Work out the finished part from the listing and answer in its coordinate system (mm). Face numbers are marked on the shaded views. Coordinates: 2 decimals unless noted, no trailing zeros. Write each loop counter-clockwise with the first axis right and the second up, starting at its lowest first coordinate (ties: lowest second). Pieces come first, ordered by that corner, then holes. Notation, with made-up numbers: (-28, 70) - (14, 70) arc R20 cw to (14, 91) - close; hole circle Ø6 at (52.25, 85). An arc over 180 degrees is marked (long way). One line per item, written item: value.
Autodesk Inventor part; units mm, degrees
ref_plane "center_point_XY" through (4.5, 0, 0) normal (1, 0, 0) x (0, 0, -1)
ref_plane "center_point_YZ" through (4.5, 0, 0) normal (0, 0, -1) x (0, 1, 0)
ref_plane "center_point_ZX" through (4.5, 0, 0) normal (0, 1, 0) x (1, 0, 0)
sketch "Sketch_1" plane through (0, 0, 0) normal (0, 0, 1) x (1, 0, 0)
  line L0 (9, 0) -> (0, 0)
  arc A0 (0, 5.6) -> (0.6, 5) centre (0.6, 5.6) ccw
  line L1 (0.6, 5) -> (8.4, 5)
  arc A1 (8.4, 5) -> (9, 5.6) centre (8.4, 5.6) ccw
  line L2 (9, 5.6) -> (9, 8.15)
  line L3 (9, 8.15) -> (8.567, 8.15)
  line L4 (8.567, 8.15) -> (8.567, 12.45)
  line L5 (8.567, 12.45) -> (9, 12.45)
  line L6 (9, 12.45) -> (9, 14.4)
  arc A2 (9, 14.4) -> (8.4, 15) centre (8.4, 14.4) ccw
  line L7 (8.4, 15) -> (0.6, 15)
  arc A3 (0.6, 15) -> (0, 14.4) centre (0.6, 14.4) ccw
  line L8 (0, 14.4) -> (0, 12.45)
  line L9 (0, 12.45) -> (0.433, 12.45)
  line L10 (0.433, 12.45) -> (0.433, 8.15)
  line L11 (0.433, 8.15) -> (0, 8.15)
  line L12 (0, 8.15) -> (0, 5.6)
revolve "Revolution1" add sketch "Sketch_1" angle 360 about axis through (9, 0, 0) along (1, 0, 0)
ref_plane "center_point_XY" through (4.5, 0, 0) normal (1, 0, 0) x (0, 0, -1)
ref_plane "center_point_YZ" through (4.5, 0, 0) normal (0, 0, -1) x (0, 1, 0)
ref_plane "center_point_ZX" through (4.5, 0, 0) normal (0, 1, 0) x (1, 0, 0)
ref_plane "to_housing_XY" through (0, 0, 0) normal (1, 0, 0) x (0, 0, -1)
ref_plane "to_housing_YZ" through (0, 0, 0) normal (0, 0, -1) x (0, 1, 0)
ref_plane "to_housing_ZX" through (0, 0, 0) normal (0, 1, 0) x (1, 0, 0)
ref_plane "to_ring_XY" through (8.134, 0, 0) normal (1, 0, 0) x (0, 0, -1)
ref_plane "to_ring_YZ" through (8.134, 0, 0) normal (0, 0, -1) x (0, 1, 0)
ref_plane "to_ring_ZX" through (8.134, 0, 0) normal (0, 1, 0) x (1, 0, 0)
properties part number "bearing_6200"
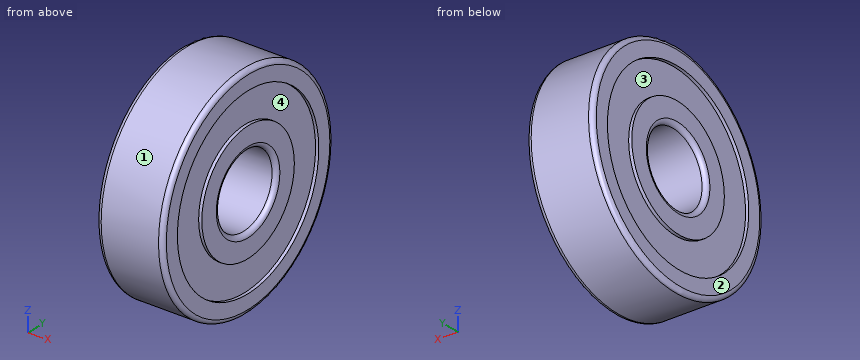
Item 1: Determine the mould class of the marked faces 1, 2, 3 and 4 for opening direction Z: +Z half, -Z half, draft (parallel to the pull), parting line (faces both ways), or undercut.
Evaluation:
face 1: parting line
face 2: draft
face 3: undercut
face 4: undercut
Item 2: Consider probe 1 along Z at (x, y) = (6.25, 0); probe 2 along Z at (x, y) = (0.1, 0); probe 3 along Y at (x, z) = (3.25, -3). Determine where each line is inside the solid, lowest interval first.
Evaluation:
probe 1: z = -15 to -5, 5 to 15
probe 2: z = -14.73 to -12.45, -8.15 to -5.27, 5.27 to 8.15, 12.45 to 14.73
probe 3: y = -14.7 to -4, 4 to 14.7
Item 3: Section C-C, the plane x = 7.75 is taken. Determine the outline of the cut face in (y, z).
Evaluation:
outline: circle Ø30 at (0, 0); hole circle Ø10 at (0, 0)
Item 4: Given pin 1 (2 mm diameter, centred on x = 6.5, z = 11, fed in from +Y); pin 2 (5 mm diameter, centred on x = 6.5, y = 7.5, fed in from +Z); pin 3 (4 mm diameter, centred on x = 1, z = 7.5, fed in from -Y), each flat-ended and moving along its own axis, determine where each tip first touches the part or whether it passes through.
Evaluation:
pin 1: stops at y = 11.18
pin 2: stops at z = 14.14
pin 3: stops at y = -13.96
